Work out the finished part from the listing and answer in its coordinate system (mm). A direction names the side the tool comes from. Coordinates: 2 decimals unless noted, no trailing zeros. Write each loop counter-clockwise with the first axis right and the second up, starting at its lowest first coordinate (ties: lowest second). Pieces come first, ordered by that corner, then holes. Notation, with made-up numbers: (37.25, 22.5) - (95.25, 22.5) arc R19 ccw to (95.25, 46.5) - close; hole circle Ø11 at (2.5, 50.25). An arc over 180 degrees is marked (long way). Use one line per item in the form item = value. Start each with the question number.
Item 1: Determine the mould class of faces 3 (the cylindrical face through (-68.62, -33.43, 32.19)), 4 (the cylindrical face through (-54.7, -6.44, 21.75)), 5 (the flat face through (-64, -127, 32)) for opening direction Y: released by +Y, released by -Y, zero draft, split by the parting line, or undercut.
Item 2: A cutting plane is placed at D-D (y = -88.9). Write down the section's boundary in (x, z) (3 decimals), then the cut area to 3 significant figures.
Item 3: A cutting plane is placed at C-C (z = 7). Write down the section's boundary in (x, y) (3 decimals).
Item 4: For faces 1 (the cylindrical face through (-59.1, -80.45, -6.26)), 2 (the flat face through (-64, -89, -12.7)), determine the directions among +Z, -Z, +X, -X, +Y, -Y from which every point of the face is accessible in a straight line to the end or side of a thin tool.
Item 5: Given pin 1 (1.5 mm diameter, centred on x = -31.5, y = -24.5, fed in from -Z); pin 2 (3 mm diameter, centred on x = -58, z = 22, fed in from +Y), each flat-ended and moving along its own axis, determine where each tip first touches the part or whether it passes through.
Item 6: A cutting plane is placed at A-A (y = -25.4). Write down the section's boundary in (x, z) (3 decimals), then the cut area to 3 significant figures.
Item 7: A cutting plane is placed at B-B (x = -63.5). Write down the section's boundary in (y, z) (3 decimals).
Item 8: Consider probe 1 along X at (y, z) = (-10, 25.4) (3 decimals); probe 2 along Z at (x, y) = (-30, -85); probe 3 along Z at (x, y) = (-63.5, -8) (3 decimals). Determine where each line is inside the solid, lowest interval first.
from build123d import *

# Parameters (mm, degrees)
F0_W     = 127
F0_H     = 63.5
F1_DEPTH = 127
F3_D     = 19.05
F4_R     = 9.525
F5_DEPTH = 12.7
F7_D     = 19.05
F7_DEPTH = 12.7
F7_TIP   = 5.7231973962


with BuildPart() as f1:
    # F0 (on Front) → F1 (new body)
    with BuildSketch(Plane.XZ):
        with Locations((-63.5, 31.75)):
            Rectangle(F0_W, F0_H)
    extrude(amount=F1_DEPTH)

    # F3 (through all)
    with Locations(Plane(origin=(0, 0, 0), x_dir=(1, 0, 0), z_dir=(0, 0, -1))):
        with Locations((-63.5, 25.4)):
            Hole(F3_D / 2)

    # F4 (on face) → F5 (join)
    with BuildSketch(Plane(origin=(0, 0, 0), x_dir=(1, 0, 0), z_dir=(0, 0, -1))):
        with Locations((-63.5, 88.9)):
            Circle(F4_R)
    extrude(amount=F5_DEPTH)

    # F7
    with Locations(Plane(origin=(0, 0, 0), x_dir=(-1, 0, 0), z_dir=(0, 1, 0))):
        with Locations((63.5, 25.4)):
            Hole(F7_D / 2, depth=F7_DEPTH)
            with Locations((0, 0, -(F7_DEPTH + F7_TIP / 2))):  # 118° drill point
                Cone(0, F7_D / 2, F7_TIP, mode=Mode.SUBTRACT)


solid = f1.part
Answer:
q1.face_3 = undercut
q1.face_4 = zero draft
q1.face_5 = released by -Y
q2.outline = (-127, 0) - (-73.025, 0) - (-73.025, -12.7) - (-53.975, -12.7) - (-53.975, 0) - (0, 0) - (0, 63.5) - (-127, 63.5) - close
q2.area = 8,310 mm²
q3.outline = (-127, -127) - (0, -127) - (0, 0) - (-127, 0) - close; hole circle Ø19.05 at (-63.5, -25.4)
q4.face_1 = -Z
q4.face_2 = -Z, +X, -X, +Y, -Y
q5.pin_1 = 0
q5.pin_2 = -13.64
q6.outline = (-127, 0) - (-73.025, 0) - (-73.025, 63.5) - (-127, 63.5) - close; (-53.975, 0) - (0, 0) - (0, 63.5) - (-53.975, 63.5) - close
q6.area = 6,850 mm²
q7.outline = (-127, 0) - (-98.425, 0) - (-98.425, -12.7) - (-79.375, -12.7) - (-79.375, 0) - (-34.925, 0) - (-34.925, 63.5) - (-127, 63.5) - close; (-15.875, 0) - (0, 0) - (0, 15.875) - (-12.7, 15.875) - (-15.875, 21.159) - close; (-15.875, 29.641) - (-12.7, 34.925) - (0, 34.925) - (0, 63.5) - (-15.875, 63.5) - close
q8.probe_1 = -127 to -73.025, -53.975 to 0
q8.probe_2 = 0 to 63.5
q8.probe_3 = 0 to 15.875, 34.925 to 63.5
